from build123d import *

# Parameters (mm, degrees)
SKETCH_1_W          = 6
SKETCH_1_H          = 30
EXTRUDE_1_DEPTH     = 177
SKETCH_2_R          = 22.5
EXTRUDE_2_DEPTH     = 6
SKETCH_3_R          = 13
CUT_EXTRUDE_1_DEPTH = 182.028312703
HOLE_WIZARD_M32_D   = 3.4
HOLE_WIZARD_M41_D   = 4.5
EXTRUDE_3_DEPTH     = 6
HOLE_WIZARD_M31_D   = 3.4
SKETCH_14_W         = 45
SKETCH_14_H         = 6
CUT_EXTRUDE_2_DEPTH = 1
SKETCH_15_W         = 30
SKETCH_15_H         = 26.9754548
CUT_EXTRUDE_3_DEPTH = 6
FILLET_1_R          = 4
CUT_EXTRUDE_4_DEPTH = 155.756628816
FILLET_3_R          = 2


with BuildPart() as part:
    # Эскиз1 → Бобышка-Вытянуть1 (new body)
    with BuildSketch(Plane(origin=(0, 0, 0), x_dir=(1, 0, 0), z_dir=(0, 1, 0))):
        with Locations((3, -15)):
            Rectangle(SKETCH_1_W, SKETCH_1_H)
    extrude(amount=EXTRUDE_1_DEPTH)

    # Эскиз2 → Бобышка-Вытянуть2 (add)
    with BuildSketch(Plane.ZY):
        with Locations((15, 105)):
            Circle(SKETCH_2_R)
    extrude(amount=-EXTRUDE_2_DEPTH)

    # Эскиз3 → Вырез-Вытянуть1 (cut, through all)
    with BuildSketch(Plane.ZY):
        with Locations((15, 105)):
            Circle(SKETCH_3_R)
    extrude(amount=-CUT_EXTRUDE_1_DEPTH, mode=Mode.SUBTRACT)

    # Отверстие с зазором M32 (through all)
    with Locations(Plane(origin=(6, -25.024735225, 7.262908886), x_dir=(0, 0, 1), z_dir=(1, 0, 0))):
        with Locations((-11.512908886, -130.024735225), (7.737091114, -110.774735225), (26.987091114, -130.024735225), (7.737091114, -149.274735225)):
            Hole(HOLE_WIZARD_M32_D / 2)

    # Отверстие с зазором M41 (through all)
    with Locations(Plane(origin=(6, 0, 0), x_dir=(0, 0, -1), z_dir=(1, 0, 0))):
        with Locations((-26, 146), (-4, 146), (-4, 64), (-26, 64)):
            Hole(HOLE_WIZARD_M41_D / 2)

    # Эскиз11 → Бобышка-Вытянуть3 (add)
    with BuildSketch(Plane(origin=(6, 0, 0), x_dir=(0, 0, -1), z_dir=(1, 0, 0))):
        Polygon((0, 18.990381057), (7.5, 6), (7.5, 0), (-37.5, 0), (-37.5, 6), (-30, 18.990381057), align=None)
    extrude(amount=-EXTRUDE_3_DEPTH)

    # Отверстие с зазором M31 (through all)
    with Locations(Plane(origin=(6, 0, 0), x_dir=(0, 0, -1), z_dir=(1, 0, 0))):
        with Locations((-28.5, 3), (-19.5, 3), (-10.5, 3), (-1.5, 3)):
            Hole(HOLE_WIZARD_M31_D / 2)

    # Эскиз14 → Вырез-Вытянуть2 (cut)
    with BuildSketch(Plane(origin=(6, 0, 0), x_dir=(0, 0, -1), z_dir=(1, 0, 0))):
        with Locations((-15, 3)):
            Rectangle(SKETCH_14_W, SKETCH_14_H)
    extrude(amount=-CUT_EXTRUDE_2_DEPTH, mode=Mode.SUBTRACT)

    # Эскиз15 → Вырез-Вытянуть3 (cut)
    with BuildSketch(Plane(origin=(6, 0, 0), x_dir=(0, 0, -1), z_dir=(1, 0, 0))):
        with Locations((-15, 163.5122726)):
            Rectangle(SKETCH_15_W, SKETCH_15_H)
    extrude(amount=-CUT_EXTRUDE_3_DEPTH, mode=Mode.SUBTRACT)

    # Скругление1
    fillet_1_edges = [part.edges().sort_by_distance(p)[0] for p in [
        (3, 150.0245452, 30),
        (3, 150.0245452, 0),
    ]]
    fillet(fillet_1_edges, radius=FILLET_1_R)

    # Эскиз16 → Вырез-Вытянуть4 (cut, through all)
    with BuildSketch(Plane.ZY):
        with BuildLine():
            Line((4, 136.794449257), (4, 124.627786426))
            ThreePointArc((4, 124.627786426), (8.352708916, 126.495662847), (13, 127.410934831))
            Line((13, 127.410934831), (13, 133.518717149))
            Line((13, 133.518717149), (4, 136.794449257))
        make_face()
        with BuildLine():
            Line((26, 136.794449257), (26, 124.627786426))
            ThreePointArc((26, 124.627786426), (21.647291084, 126.495662847), (17, 127.410934831))
            Line((17, 127.410934831), (17, 133.518717149))
            Line((17, 133.518717149), (26, 136.794449257))
        make_face()
        Polygon((7.538207724, 139.763358053), (15, 137.04748777), (22.461792276, 139.763358053), (15, 146.0245452), align=None)
        with BuildLine():
            Line((13, 76.479065169), (13, 82.589065169))
            ThreePointArc((13, 82.589065169), (8.352708916, 83.504337153), (4, 85.372213574))
            Line((4, 85.372213574), (4, 73.203333061))
            Line((4, 73.203333061), (13, 76.479065169))
        make_face()
        with BuildLine():
            Line((17, 76.479065169), (17, 82.589065169))
            ThreePointArc((17, 82.589065169), (21.647291084, 83.504337153), (26, 85.372213574))
            Line((26, 85.372213574), (26, 73.203333061))
            Line((26, 73.203333061), (17, 76.479065169))
        make_face()
        Polygon((7.560453217, 70.242520962), (15, 72.950294548), (22.439546783, 70.242520962), (15, 64), align=None)
        Polygon((26, 53.881197846), (26, 28.477786002), (4, 41.179491924), align=None)
        Polygon((4, 58.5), (26, 58.5), (4, 45.798294078), align=None)
        Polygon((4, 36.560689771), (26, 23.858983849), (4, 11.157277926), align=None)
        Polygon((11.72758664, 11), (26, 19.240181695), (26, 11), align=None)
    extrude(amount=-CUT_EXTRUDE_4_DEPTH, mode=Mode.SUBTRACT)

    # Скругление3
    fillet_3_edges = [part.edges().sort_by_distance(p)[0] for p in [
        (3, 88.229490169, 0),
        (3, 121.770509831, 0),
        (3, 127.410934831, 13),
        (3, 124.627786426, 4),
        (3, 136.794449257, 4),
        (3, 133.518717149, 13),
        (3, 88.229490169, 30),
        (3, 124.627786426, 26),
        (3, 121.770509831, 30),
        (3, 127.410934831, 17),
        (3, 133.518717149, 17),
        (3, 136.794449257, 26),
        (3, 146.0245452, 15),
        (3, 139.763358053, 22.461792276),
        (3, 137.04748777, 15),
        (3, 139.763358053, 7.538207724),
        (3, 76.479065169, 13),
        (3, 73.203333061, 4),
        (3, 85.372213574, 4),
        (3, 82.589065169, 13),
        (3, 73.203333061, 26),
        (3, 76.479065169, 17),
        (3, 82.589065169, 17),
        (3, 85.372213574, 26),
        (3, 64, 15),
        (3, 70.242520962, 7.560453217),
        (3, 72.950294548, 15),
        (3, 70.242520962, 22.439546783),
        (3, 41.179491924, 4),
        (3, 53.881197846, 26),
        (3, 28.477786002, 26),
        (3, 45.798294078, 4),
        (3, 58.5, 4),
        (3, 58.5, 26),
        (3, 11.157277926, 4),
        (3, 36.560689771, 4),
        (3, 23.858983849, 26),
        (3, 11, 26),
        (3, 11, 11.72758664),
        (3, 19.240181695, 26),
        (3, 18.990381057, 30),
        (3, 18.990381057, 0),
    ]]
    fillet(fillet_3_edges, radius=FILLET_3_R)


solid = part.part
CAD build for the part. Positions are in the model's coordinates, mm. A direction names the side the tool comes from. Round coordinates to 2 decimals unless told otherwise and drop trailing zeros. Order: outer loops, then holes, each group sorted by start corner. A loop starts at its lowest first (then second) coordinate and runs counter-clockwise, first axis right, second up. Notation, with made-up numbers: (85, 65.25) -> (112, 65.25) arc R24 ccw to (112, 88.25) -> close; hole circle Ø5 at (55, -24.5). An arc over 180 degrees is marked (long way). Write each question's results on one line, items separated by ' | '.
1. Flat gauge pins, fed straight in: P1, Ø3, axis at x = 4.5, y = 112.5, coming from the +Z side; P2, Ø3, axis at x = 4, y = 39, coming from the -Z side; P3, Ø3, axis at x = 2.5, y = 66.5, coming from the +Z side. Where does each tip first touch, or does it go through?
Findings below:
P1: stops at z = 36.69 | P2: stops at z = 0 | P3: stops at z = 30
2. 3-axis set-ups, long thin cutter, end or side, ignore diameter. For faces 1 (the face through (3, 105.3, -7.5)), 2 (the face through (3, 79, 13)): which of +Z, -Z, +X, -X, +Y, -Y reach the whole face in a straight line?
Findings below:
face 1: -Z, +X, -X | face 2: +X, -X
3. Cut at A-A (y = 3). Give the cut face in (x, z), plus the area to 3 significant figures.
Findings below:
outline: (0, -7.5) -> (5, -7.5) -> (5, -0.2) -> (0, -0.2) -> close; (0, 3.2) -> (5, 3.2) -> (5, 8.8) -> (0, 8.8) -> close; (0, 12.2) -> (5, 12.2) -> (5, 17.8) -> (0, 17.8) -> close; (0, 21.2) -> (5, 21.2) -> (5, 26.8) -> (0, 26.8) -> close; (0, 30.2) -> (5, 30.2) -> (5, 37.5) -> (0, 37.5) -> close | area: 157 mm²
4. Wall check: line 1 along Z through (x, y) = (2.35, 146); line 2 along Z through (x, y) = (1.3, 124.25); line 3 along Y through (x, z) = (2.25, -4.25). Give the ranges that are in metal, low to high. Write a range as [from, to].
Findings below:
line 1: z = [0, 1.75], [6.25, 23.75], [28.25, 30] | line 2: z = [0, 13.3], [16.7, 30] | line 3: y = [0, 11.63], [93.35, 103.3], [106.7, 116.65]
5. Cut at B-B (y = 85.75). Give the cut face in (x, z), plus the area to 3 significant figures.
Findings below:
outline: (0, 0) -> (6, 0) -> (6, 13.3) -> (0, 13.3) -> close; (0, 16.7) -> (6, 16.7) -> (6, 30) -> (0, 30) -> close | area: 160 mm²
6. Cut at C-C (y = 105). Give the cut face in (x, z), plus the area to 3 significant figures.
Findings below:
outline: (0, -7.5) -> (6, -7.5) -> (6, -5.95) -> (0, -5.95) -> close; (0, -2.55) -> (6, -2.55) -> (6, 2) -> (0, 2) -> close; (0, 28) -> (6, 28) -> (6, 32.55) -> (0, 32.55) -> close; (0, 35.95) -> (6, 35.95) -> (6, 37.5) -> (0, 37.5) -> close | area: 73.2 mm²
7. Pull direction Y, two halves, no side cores. Call faces 3 (the face through (3, 150.025, 15)), 4 (the face through (3, 134, 0)), 5 (the face through (3, 66.6, 18.1)): pulls with the +Y half, pulls with the -Y half, needs draft (parallel to the pull), parting line crosses it, or undercut.
Findings below:
face 3: pulls with the +Y half | face 4: needs draft | face 5: undercut
8. Cut at D-D (x = 2.25). Count the separate pieces of the cut face and the enclosed holes in it, plus the area to 3 significant figures.
Findings below:
separate pieces: 1 | enclosed holes: 23 | area: 3,230 mm²
